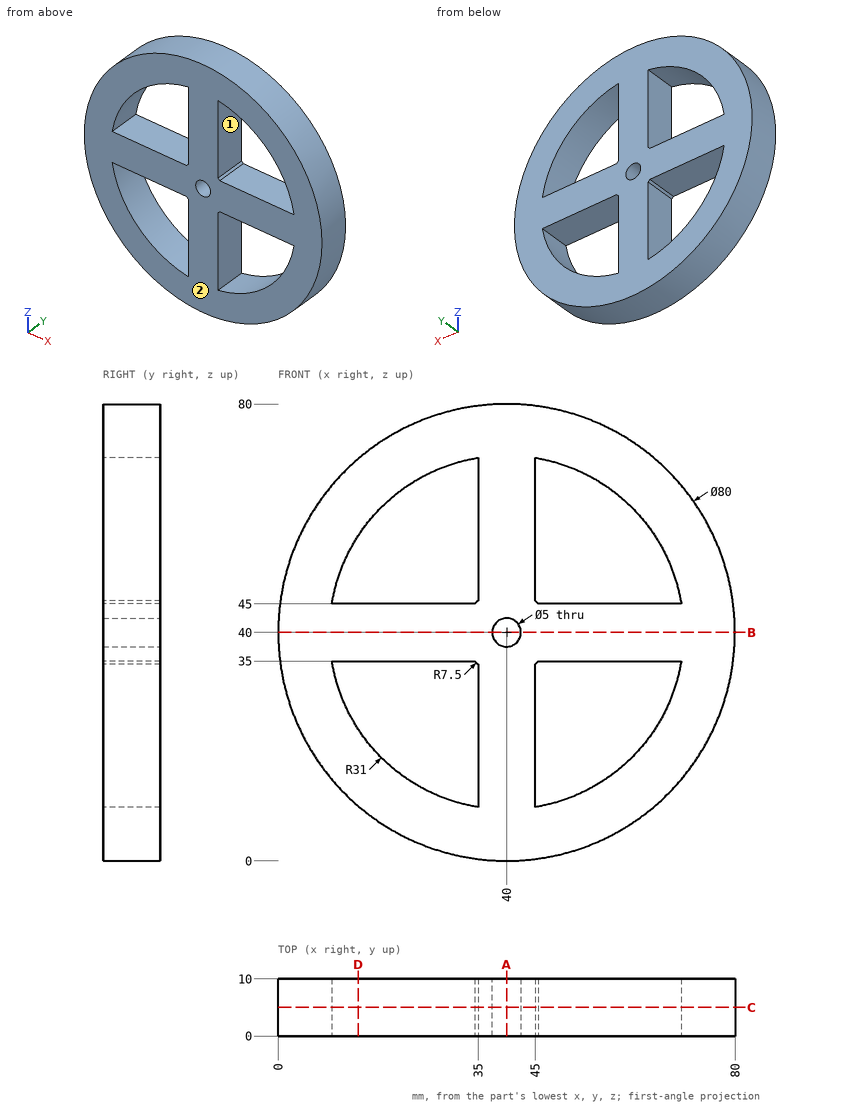
Geometry check sheet. Reference: drawing and pictorial views, mm from the part's lowest x, y, z. A direction names the side the tool comes from. Round coordinates to 2 decimals unless told otherwise and drop trailing zeros. Loops run counter-clockwise (first coordinate to the right, second up) from the corner with the lowest first, then second, coordinate; pieces in that order, holes last.
1. Scan lines: probe 1 along X at (y, z) = (9.25, 61.5); probe 2 along X at (y, z) = (3, 19); probe 3 along Z at (x, y) = (40, 2). Record each from-to range of solid material in increasing order.
2. Gauge pin test, flat ends, axial feed: pin 1 Ø3 at (x, y) = (59.5, 4.5) entering from -Z; pin 2 Ø5 at (x, y) = (21, 1.5) entering from -Z; pin 3 Ø3 at (x, y) = (57, 6) entering from +Z; pin 4 Ø4 at (x, z) = (40, 40) entering from -Y. Record the tip position at first contact, or that the pin passes through.
3. Set-up check for the marked faces 1 and 2: record each of +Z, -Z, +X, -X, +Y, -Y from which the full face is reachable in a straight line by a thin tool's end or side.
4. Sectioned sample at B-B on z = 40. Record the boundary of the cut face in (x, y).
5. Sectioned sample at C-C on y = 5. Record the boundary of the cut face in (x, z).
6. Sectioned sample at A-A on x = 40. Record the boundary of the cut face in (y, z), and give its area (3 significant figures).
7. Sectioned sample at D-D on x = 14. Record the boundary of the cut face in (y, z).
Recorded:
1. probe 1: x = 6.27 to 17.67, 35 to 45, 62.33 to 73.73
1. probe 2: x = 5.96 to 17.2, 35 to 45, 62.8 to 74.04
1. probe 3: z = 0 to 37.5, 42.5 to 80
2. pin 1: stops at z = 4.28
2. pin 2: stops at z = 3.56
2. pin 3: stops at z = 76.87
2. pin 4: passes through
3. face 1: +Y, -Y
3. face 2: +Z, -Z, +X, -X, -Y
4. outline: (0, 0) - (37.5, 0) - (37.5, 10) - (0, 10) - close; (42.5, 0) - (80, 0) - (80, 10) - (42.5, 10) - close
5. outline: circle Ø80 at (40, 40); hole (9.41, 35) arc R31 ccw to (35, 9.41) - (35, 34.41) arc R7.5 cw to (34.41, 35) - close; hole (9.41, 45) - (34.41, 45) arc R7.5 cw to (35, 45.59) - (35, 70.59) arc R31 ccw to start; hole circle Ø5 at (40, 40); hole (45, 9.41) arc R31 ccw to (70.59, 35) - (45.59, 35) arc R7.5 cw to (45, 34.41) - close; hole (45, 45.59) arc R7.5 cw to (45.59, 45) - (70.59, 45) arc R31 ccw to (45, 70.59) - close
6. outline: (0, 0) - (10, 0) - (10, 37.5) - (0, 37.5) - close; (0, 42.5) - (10, 42.5) - (10, 80) - (0, 80) - close
6. area: 750 mm2
7. outline: (0, 9.6) - (10, 9.6) - (10, 23.12) - (0, 23.12) - close; (0, 35) - (10, 35) - (10, 45) - (0, 45) - close; (0, 56.88) - (10, 56.88) - (10, 70.4) - (0, 70.4) - close
